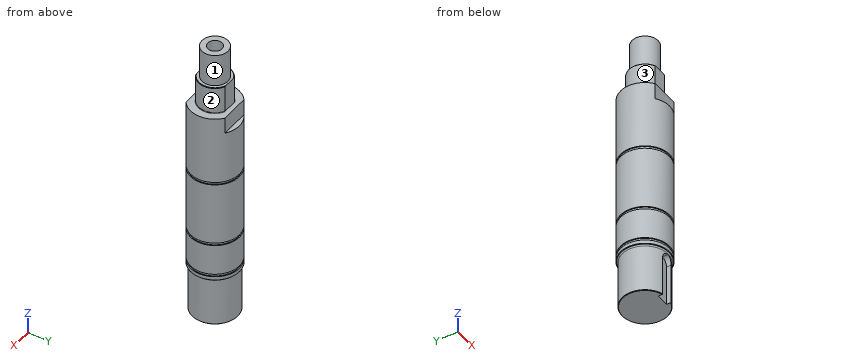
from build123d import *

# Parameters (mm, degrees)
F2_SIZE   = 0.29999
F4_DEPTH  = 28.8
F5_R      = 3.9999
F6_W      = 16.3141209632
F6_H      = 1.5053940788
F7_DEPTH  = 16.6
F8_W      = 11.3712083548
F8_H      = 5.6990628242
F9_DEPTH  = 10
F11_D     = 8.8
F11_DEPTH = 15
F11_TIP   = 2.6437867237


# Not quite as in the source:
# - a fillet or chamfer is up to 0.001 mm smaller than in the source, because OpenCascade refuses the exact size


with BuildPart() as f1:
    # F0 (on Front) → F1 (revolve)
    with BuildSketch(Plane.XZ):
        with BuildLine():
            Line((-14, 0), (0, 0))
            Line((0, 0), (0, 173.8))
            Line((0, 173.8), (-8, 173.8))
            Line((-8, 173.8), (-8, 153.8))
            Line((-8, 153.8), (-10, 153.8))
            Line((-10, 153.8), (-10, 137.5))
            ThreePointArc((-10, 137.5), (-10.0878679656, 137.2878679656), (-10.3, 137.2))
            Line((-10.3, 137.2), (-15, 137.2))
            Line((-15, 137.2), (-15, 137))
            Line((-15, 137), (-15, 136.8790119886))
            Line((-15, 136.8790119886), (-15, 95.1))
            Line((-15, 95.1), (-14.4, 95.1))
            Line((-14.4, 95.1), (-14.4, 93.5))
            Line((-14.4, 93.5), (-15, 93.5))
            Line((-15, 93.5), (-15, 54.8))
            Line((-15, 54.8), (-14.4, 54.8))
            Line((-14.4, 54.8), (-14.4, 53.2))
            Line((-14.4, 53.2), (-15, 53.2))
            Line((-15, 53.2), (-15, 34.1))
            Line((-15, 34.1), (-14.4, 34.1))
            Line((-14.4, 34.1), (-14.4, 32.5))
            Line((-14.4, 32.5), (-15, 32.5))
            Line((-15, 32.5), (-15, 30))
            Line((-15, 30), (-14.7, 30))
            ThreePointArc((-14.7, 30), (-14.2050252532, 29.7949747468), (-14, 29.3))
            Line((-14, 29.3), (-14, 0))
        make_face()
    revolve(axis=Axis((0, 0, 86.9), (0, 0, -1)))

    # F2 (size 0.3 in the source; OpenCascade refuses exactly that, so slightly less here)
    f2_edges = [f1.edges().sort_by_distance(p)[0] for p in [
        (15, 0, 30),
        (10, 0, 153.8),
        (14, 0, 0),
    ]]
    chamfer(f2_edges, length=F2_SIZE)

    # F3 (on face) → F4 (cut)
    with BuildSketch(Plane(origin=(0, 0, 0), x_dir=(1, 0, 0), z_dir=(0, 0, -1))):
        Polygon((4, 14), (0, 14), (-4, 14), (-4, 10.6), (0, 10.6), (4, 10.6), align=None)
    extrude(amount=-F4_DEPTH, mode=Mode.SUBTRACT)

    # F5 (radius 4 in the source; OpenCascade refuses exactly that, so slightly less here)
    f5_edges = [f1.edges().sort_by_distance(p)[0] for p in [
        (4, -12.008204, 28.8),
        (-4, -12.008204, 28.8),
    ]]
    fillet(f5_edges, radius=F5_R)

    # F6 (on face) → F7 (cut, through all)
    with BuildSketch(Plane.XY.offset(153.8)):
        with Locations((-8.1570604816, -9.7526970394)):
            Rectangle(F6_W, F6_H)
        with Locations((8.1570604816, -9.7526970394)):
            Rectangle(F6_W, F6_H)
        Polygon((-16.3141209632, 9), (0, 9), (16.3141209632, 9), (16.3141209632, 10.5053940788), (0, 10.5053940788), (-16.3141209632, 10.5053940788), align=None)
    extrude(amount=-F7_DEPTH, mode=Mode.SUBTRACT)

    # F8 (on face) → F9 (cut)
    with BuildSketch(Plane.XY.offset(137.2)):
        with Locations((5.6856041774, 14.8495314121)):
            Rectangle(F8_W, F8_H)
        with Locations((-5.6856041774, 14.8495314121)):
            Rectangle(F8_W, F8_H)
        Polygon((0, -17.6990628242), (11.3712083548, -17.6990628242), (11.3712083548, -12), (0, -12), (-11.3712083548, -12), (-11.3712083548, -17.6990628242), align=None)
    extrude(amount=-F9_DEPTH, mode=Mode.SUBTRACT)

    # F11
    with Locations(Plane.XY.offset(173.8)):
        with Locations((0, 0)):
            Hole(F11_D / 2, depth=F11_DEPTH)
            with Locations((0, 0, -(F11_DEPTH + F11_TIP / 2))):  # 118° drill point
                Cone(0, F11_D / 2, F11_TIP, mode=Mode.SUBTRACT)


solid = f1.part
Could you check a few things on this model? Use its own coordinates, in mm. Face numbers are marked on the shaded views. A direction names the side the tool comes from. Round coordinates to 2 decimals unless told otherwise and drop trailing zeros. Write each loop counter-clockwise with the first axis right and the second up, starting at its lowest first coordinate (ties: lowest second). Pieces come first, ordered by that corner, then holes. Notation, with made-up numbers: (4.25, -2.75) - (21.25, -2.75) arc R16 cw to (21.25, 20.25) - close; hole circle Ø8 at (86, 44). An arc over 180 degrees is marked (long way). Put each result on its own line as item: value. Start each with the question number.
(1) I need wall thicknesses on probe 1 along X at (y, z) = (0.5, 159); probe 2 along Z at (x, y) = (-11.25, -9.75); probe 3 along Y at (x, z) = (0, 167.75). Which ranges of each line are inside material? Lowest first, please.
(2) Will these pins go through, and if not, where does the flat tip stop? pin 1 (8 mm diameter, centred on x = 0, z = 144.5, fed in from -Y); pin 2 (3 mm diameter, centred on y = -12.5, z = 12.5, fed in from +X); pin 3 (1.5 mm diameter, centred on x = -1.5, z = 52.5, fed in from -Y).
(3) I want a section at A-A, the plane z = 118.5. Please give me the cut outline in (x, y), plus the area to 3 significant figures.
(4) For the marked faces 1, 2 and 3, which set-ups out of +Z, -Z, +X, -X, +Y, -Y let a thin tool reach every point of the face, with its end or its side?
Here are the results:
1. probe 1: x = -7.98 to -4.37, 4.37 to 7.98
1. probe 2: z = 30.19 to 32.5, 34.1 to 53.2, 54.8 to 93.5, 95.1 to 137.2
1. probe 3: y = -8 to -4.4, 4.4 to 8
2. pin 1: stops at y = -9
2. pin 2: stops at x = 8.66
2. pin 3: stops at y = -14.98
3. outline: circle Ø30 at (0, 0)
3. area: 707 mm^2
4. face 1: +Z
4. face 2: +Z, +X
4. face 3: +Z, -X
